from build123d import *

# Parameters (mm, degrees)
F1_DEPTH = 2438.4
F2_R     = 82.55
F3_DEPTH = 25.4


with BuildPart() as f1:
    # F0 (on Top) → F1 (new body)
    with BuildSketch(Plane.XY):
        Polygon((-609.6, 3.175), (-609.6, -6.35), (609.6, -6.35), (609.6, 6.35), (-571.5, 6.35), align=None)
    extrude(amount=F1_DEPTH)

    # F2 (on face) → F3 (cut)
    with BuildSketch(Plane.XZ.offset(6.35)):
        with Locations((-241.3, 1041.4)):
            Circle(F2_R)
    extrude(amount=-F3_DEPTH, mode=Mode.SUBTRACT)


solid = f1.part
Source: CAD feature listing. Evaluate the final solid. Frame: model axes, mm. Round coordinates to 2 decimals unless told otherwise and drop trailing zeros. Write each loop counter-clockwise with the first axis right and the second up, starting at its lowest first coordinate (ties: lowest second). Pieces come first, ordered by that corner, then holes. Notation, with made-up numbers: M 46.25,12 L 50.25,12 A27 cw 50.25,45 Z; hole C 72,41 d3. An arc over 180 degrees is marked long. One line per item, written item: value. Start each with the question number.
Item 1: Mould query, pull axis Z, two halves, no side actions, for faces 1 (the cylindrical face through (-196.922, -0.089, 1111.006)), 2 (the flat face through (27, 6.35, 1202)). Classes: pulls with the +Z half, pulls with the -Z half, needs draft (parallel to the pull), parting line crosses it, or undercut.
Item 2: Section query A-A (x = -241.3). Return the cut outline in (y, z).
Item 3: Section query B-B (z = 1041.4). Return the cut outline in (x, y) (3 decimals), plus the area to 3 significant figures.
Item 4: Ray query, L1, parallel to Z at x = -241.3, y = -1; L2, parallel to X at y = -2.75, z = 971.5; L3, parallel to Z at x = -267.5, y = 5.25. Return the intervals inside material, ascending. Write a range as from..to.
Result set:
1. face 1: undercut
1. face 2: needs draft
2. outline: M -6.35,0 L 6.35,0 L 6.35,958.85 L -6.35,958.85 Z; M -6.35,1123.95 L 6.35,1123.95 L 6.35,2438.4 L -6.35,2438.4 Z
3. outline: M -609.6,-6.35 L -323.85,-6.35 L -323.85,6.35 L -571.5,6.35 L -609.6,3.175 Z; M -158.75,-6.35 L 609.6,-6.35 L 609.6,6.35 L -158.75,6.35 Z
3. area: 13,300 mm²
4. L1: z = 0..958.85, 1123.95..2438.4
4. L2: x = -609.6..-285.21, -197.39..609.6
4. L3: z = 0..963.12, 1119.68..2438.4
